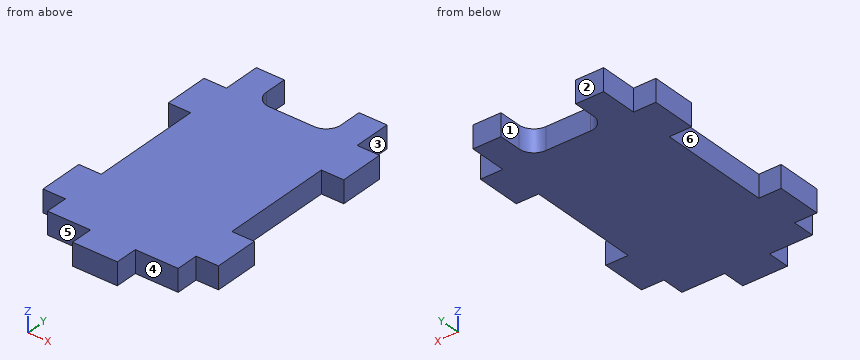
from build123d import *

# Parameters (mm, degrees)
SKETCH1_W           = 6
SKETCH1_H           = 6
BOSS_EXTRUDE1_DEPTH = 6
SKETCH1_3_W         = 6
SKETCH1_3_H         = 12
BOSS_EXTRUDE2_DEPTH = 6
FILLET2_R           = 4


with BuildPart() as part:
    # Sketch1 → Boss-Extrude1 (new body)
    with BuildSketch(Plane.XY):
        Polygon((-17.5, 35), (-17.5, -35), (0, 0), align=None)
        Polygon((-10, 35), (-17.5, 35), (0, 0), (17.5, 35), (10, 35), (10, 25), (-10, 25), align=None)
        Polygon((0, 0), (17.5, -35), (17.5, -29), (17.5, -17), (17.5, 13), (17.5, 25), (17.5, 35), align=None)
        Polygon((-6, -35), (0, -35), (6, -35), (17.5, -35), (0, 0), (-17.5, -35), align=None)
        with Locations((3, -38)):
            Rectangle(SKETCH1_W, SKETCH1_H)
        with Locations((-3, -38)):
            Rectangle(SKETCH1_W, SKETCH1_H)
    extrude(amount=-BOSS_EXTRUDE1_DEPTH)

    # Sketch1<3> → Boss-Extrude2 (add)
    with BuildSketch(Plane.XY):
        with Locations((20.5, 19)):
            Rectangle(SKETCH1_3_W, SKETCH1_3_H)
        with Locations((20.5, -23)):
            Rectangle(SKETCH1_3_W, SKETCH1_3_H)
    boss_extrude2 = extrude(amount=-BOSS_EXTRUDE2_DEPTH)

    # Mirror1: Boss-Extrude2 across plane
    add(boss_extrude2.mirror(Plane(origin=(0, 0, 0), x_dir=(0, 0, 1), z_dir=(1, 0, 0))))

    # Fillet2
    fillet2_edges = [part.edges().sort_by_distance(p)[0] for p in [
        (-10, 25, -3),
        (10, 25, -3),
    ]]
    fillet(fillet2_edges, radius=FILLET2_R)


solid = part.part
Work out the finished part from the listing and answer in its coordinate system (mm). Face numbers are marked on the shaded views. A direction names the side the tool comes from. Coordinates: 2 decimals unless noted, no trailing zeros. Loops run counter-clockwise (first coordinate to the right, second up) from the corner with the lowest first, then second, coordinate; pieces in that order, holes last. Notation, with made-up numbers: (-12.5, -16) -> (24.5, -16) arc R8 ccw to (24.5, -3) -> close; hole circle Ø8 at (-33, -0.5). An arc over 180 degrees is marked (long way). Answer as CSV lines item,"result".
1) The part is cut by section C-C (y = -10). Give the vertices of the cut face in (x, z), and give its area (3 significant figures).
A:
outline,"(-17.5, -6) -> (17.5, -6) -> (17.5, 0) -> (-17.5, 0) -> close"
area,"210 mm²"
2) Flat-ended cylindrical pins translate along their axes: pin 1 (3 mm diameter, centred on y = -31.5, z = -2.5, fed in from +X); pin 2 (1.5 mm diameter, centred on x = 17, z = -1, fed in from -Y); pin 3 (1.8 mm diameter, centred on y = 31.5, z = -2, fed in from -X); pin 4 (5 mm diameter, centred on x = -9.5, y = -12.5, fed in from +Z). Find the tip coordinate at first contact, or state that the pin passes through.
A:
pin 1,"stops at x = 17.5"
pin 2,"stops at y = -35"
pin 3,"stops at x = -17.5"
pin 4,"stops at z = 0"
3) Straight lines are drawn through the part: probe 1 along Y at (x, z) = (-20.5, -0.25); probe 2 along X at (y, z) = (-8.5, -0.6); probe 3 along X at (y, z) = (29, -3.45). For each, find the intervals that lie inside material, in ascending order.
A:
probe 1,"y = -29 to -17, 13 to 25"
probe 2,"x = -17.5 to 17.5"
probe 3,"x = -17.5 to -10, 10 to 17.5"
4) For the marked faces 4, 5 and 6, determine the directions among +Z, -Z, +X, -X, +Y, -Y from which every point of the face is accessible in a straight line to the end or side of a thin tool.
A:
face 4,"+Z, -Z, +X, -Y"
face 5,"+Z, -Z, -X, -Y"
face 6,"+Z, -Z, -X"
5) The part is cut by section B-B (x = -13). Give the vertices of the cut face in (y, z), and give its area (3 significant figures).
A:
outline,"(-35, -6) -> (35, -6) -> (35, 0) -> (-35, 0) -> close"
area,"420 mm²"
6) For a pull along X with two mould halves and no side action, classify the marked faces 1, 2 and 3 as released by +X, released by -X, zero draft, split by the parting line, or undercut.
A:
face 1,"undercut"
face 2,"zero draft"
face 3,"released by +X"
